```python
from build123d import *

# Parameters (mm, degrees)
BOSS_EXTRUDE1_START = 12.075
SKETCH1_W           = 32.8
SKETCH1_H           = 16.2
BOSS_EXTRUDE1_DEPTH = 6.925
CUT_EXTRUDE1_START  = 6.5
SKETCH2_W           = 32.8
SKETCH2_H           = 13
CUT_EXTRUDE1_DEPTH  = 1.35
CUT_EXTRUDE2_START  = 12.025
SKETCH3_W           = 23.4
SKETCH3_H           = 13
CUT_EXTRUDE2_DEPTH  = 4.175
CUT_EXTRUDE3_START  = 17.6
SKETCH4_R           = 3.8
CUT_EXTRUDE3_DEPTH  = 1.4
CUT_EXTRUDE4_START  = 11.84
SKETCH5_R           = 0.925
CUT_EXTRUDE4_DEPTH  = 4.01


with BuildPart() as part:
    # Sketch1 → Boss-Extrude1 (new, symmetric)
    with BuildSketch(Plane(origin=(0, 0, 0), x_dir=(1, 0, 0), z_dir=(0, 1, 0)).offset(BOSS_EXTRUDE1_START)):
        Rectangle(SKETCH1_W, SKETCH1_H)
    extrude(amount=BOSS_EXTRUDE1_DEPTH, both=True)

    # Sketch2 → Cut-Extrude1 (cut, symmetric)
    with BuildSketch(Plane(origin=(0, 0, 0), x_dir=(1, 0, 0), z_dir=(0, 1, 0)).offset(CUT_EXTRUDE1_START)):
        Rectangle(SKETCH2_W, SKETCH2_H)
    extrude(amount=CUT_EXTRUDE1_DEPTH, both=True, mode=Mode.SUBTRACT)

    # Sketch3 → Cut-Extrude2 (cut, symmetric)
    with BuildSketch(Plane(origin=(0, 0, 0), x_dir=(1, 0, 0), z_dir=(0, 1, 0)).offset(CUT_EXTRUDE2_START)):
        Rectangle(SKETCH3_W, SKETCH3_H)
    extrude(amount=CUT_EXTRUDE2_DEPTH, both=True, mode=Mode.SUBTRACT)

    # Sketch4 → Cut-Extrude3 (cut, symmetric)
    with BuildSketch(Plane(origin=(0, 0, 0), x_dir=(1, 0, 0), z_dir=(0, 1, 0)).offset(CUT_EXTRUDE3_START)):
        with Locations(Location((5.5, 0, 0), (0, 0, 270))):
            Circle(SKETCH4_R)
    extrude(amount=CUT_EXTRUDE3_DEPTH, both=True, mode=Mode.SUBTRACT)

    # Sketch5 → Cut-Extrude4 (cut, symmetric)
    with BuildSketch(Plane(origin=(0, 0, 0), x_dir=(1, 0, 0), z_dir=(0, 1, 0)).offset(CUT_EXTRUDE4_START)):
        with Locations(Location((-13.75, 0, 0), (0, 0, 270))):
            Circle(SKETCH5_R)
        with Locations(Location((13.75, 0, 0), (0, 0, 270))):
            Circle(SKETCH5_R)
    extrude(amount=CUT_EXTRUDE4_DEPTH, both=True, mode=Mode.SUBTRACT)


solid = part.part
```
Input: part model. Units: mm. Frame: model coordinates. A direction names the side the tool comes from. Round coordinates to 2 decimals unless told otherwise and drop trailing zeros. Order: outer loops, then holes, each group sorted by start corner. A loop starts at its lowest first (then second) coordinate and runs counter-clockwise, first axis right, second up. Notation, with made-up numbers: (32.5, -32) - (80.5, -32) arc R16 cw to (80.5, -22) - close; hole circle Ø4 at (75, -15). An arc over 180 degrees is marked (long way). Answer in a Markdown table with one row per item.
Item 1: Section query C-C (x = -9.5). Return the cut outline in (y, z), then the cut area to 3 significant figures.
Model answer:
| item | result |
|---|---|
| outline | (5.15, -8.1) - (19, -8.1) - (19, 8.1) - (5.15, 8.1) - (5.15, 6.5) - (16.2, 6.5) - (16.2, -6.5) - (5.15, -6.5) - close |
| area | 80.7 mm² |
Item 2: Line query: line 1 (X direction, y = 9.05, z = 0) (3 decimals); line 2 (X direction, y = 8, z = 4); line 3 (X direction, y = 8.75, z = -0.5). Output: solid intervals per line, ascending.
Model answer:
| item | result |
|---|---|
| line 1 | x = -16.4 to -14.675, -12.825 to -11.7, 11.7 to 12.825, 14.675 to 16.4 |
| line 2 | x = -16.4 to -11.7, 11.7 to 16.4 |
| line 3 | x = -16.4 to -14.53, -12.97 to -11.7, 11.7 to 12.97, 14.53 to 16.4 |
Item 3: Mould query, pull axis X, two halves, no side actions, for faces 4 (the flat face through (11.7, 12, 0)), 5 (the flat face through (16.4, 14, 0)), 6 (the flat face through (0, 12, -8.1)). Classes: released by +X, released by -X, zero draft, split by the parting line, or undercut.
Model answer:
| item | result |
|---|---|
| face 4 | undercut |
| face 5 | released by +X |
| face 6 | zero draft |
Item 4: Pin query (flat end, axial travel): pin 1 (5 mm diameter, centred on x = -13.5, z = 1.5, fed in from -Y); pin 2 (3 mm diameter, centred on x = 5, z = 4, fed in from -Y); pin 3 (0.6 mm diameter, centred on x = 14, z = -0.5, fed in from -Y). Return the tip coordinate at first contact, or that it passes through.
Model answer:
| item | result |
|---|---|
| pin 1 | stops at y = 7.85 |
| pin 2 | stops at y = 16.2 |
| pin 3 | stops at y = 15.85 |
Item 5: Section query B-B (z = 0). Return the cut outline in (x, y) (3 decimals), then the cut area to 3 significant figures.
Model answer:
| item | result |
|---|---|
| outline | (-16.4, 7.85) - (-14.675, 7.85) - (-14.675, 15.85) - (-12.825, 15.85) - (-12.825, 7.85) - (-11.7, 7.85) - (-11.7, 16.2) - (1.7, 16.2) - (1.7, 19) - (-16.4, 19) - close; (9.3, 16.2) - (11.7, 16.2) - (11.7, 7.85) - (12.825, 7.85) - (12.825, 15.85) - (14.675, 15.85) - (14.675, 7.85) - (16.4, 7.85) - (16.4, 19) - (9.3, 19) - close |
| area | 119 mm² |
Item 6: Section query A-A (y = 7.5). Return the cut outline in (x, z).
Model answer:
| item | result |
|---|---|
| outline | (-16.4, -8.1) - (16.4, -8.1) - (16.4, -6.5) - (-16.4, -6.5) - close; (-16.4, 6.5) - (16.4, 6.5) - (16.4, 8.1) - (-16.4, 8.1) - close |
Item 7: Section query D-D (y = 12.5). Return the cut outline in (x, z) (3 decimals), then the cut area to 3 significant figures.
Model answer:
| item | result |
|---|---|
| outline | (-16.4, -8.1) - (16.4, -8.1) - (16.4, 8.1) - (-16.4, 8.1) - close; hole circle Ø1.85 at (-13.75, 0); hole (-11.7, -6.5) - (11.7, -6.5) - (11.7, 6.5) - (-11.7, 6.5) - close; hole circle Ø1.85 at (13.75, 0) |
| area | 222 mm² |
Item 8: Reachability of faces 1 (the flat face through (-15, 7.85, 0)), 2 (the flat face through (0, 11, -6.5)), 3 (the flat face through (0, 19, 0)) from +Z, -Z, +X, -X, +Y, -Y: full face, straight path, thin tool, end or side. Return the list, or none.
Model answer:
| item | result |
|---|---|
| face 1 | +X, -X, -Y |
| face 2 | -Y |
| face 3 | +Z, -Z, +X, -X, +Y |
